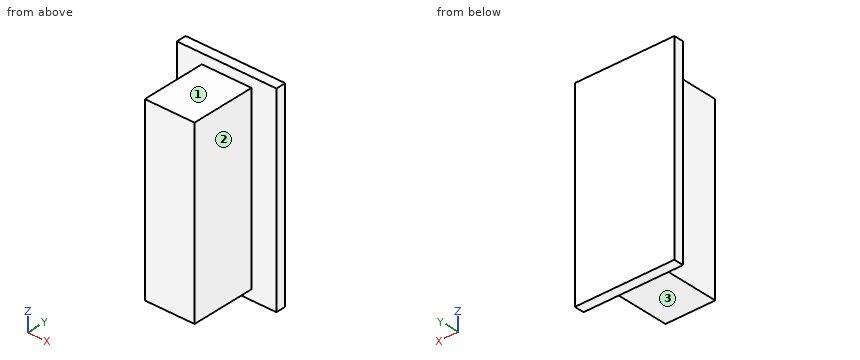
Autodesk Inventor part; units mm, degrees
ref_plane "YZ Plane" through (0, 0, 0) normal (1, 0, 0) x (0, 1, 0)
ref_plane "XZ Plane" through (0, 0, 0) normal (0, 1, 0) x (-1, 0, 0)
ref_plane "XY Plane" through (0, 0, 0) normal (0, 0, 1) x (1, 0, 0)
sketch "スケッチ1" plane through (0, 0, 0) normal (0, 1, 0) x (-1, 0, 0)
  line L0 (10, 20) -> (-10, 20)
  line L1 (-10, 20) -> (-10, -20)
  line L2 (-10, -20) -> (10, -20)
  line L3 (10, -20) -> (10, 20)
  line L4 (10, 20) -> (-10, -20) construction
  line L5 (-10, 20) -> (10, -20) construction
  line L6 (5, 18) -> (-5, 18)
  line L7 (-5, 18) -> (-5, -18)
  line L8 (-5, -18) -> (5, -18)
  line L9 (5, -18) -> (5, 18)
  line L10 (5, 18) -> (-5, -18) construction
  line L11 (-5, 18) -> (5, -18) construction
  point P0 (0, 0)
  dimension "d0" = 40
  dimension "d1" = 20
  dimension "d2" = 2
  dimension "d3" = 10
extrude "押し出し1" add sketch "スケッチ1" along normal blind 2 contours L3 L2 L1 L0 | L9 L8 L7 L6
extrude "押し出し2" add sketch "スケッチ1" against normal blind 13 contours L9 L8 L7 L6
properties part number "i2chub"
Check sheet for the modelled part. Datum: model origin and axes. Units: mm. Face numbers are marked on the shaded views. A direction names the side the tool comes from. Round coordinates to 2 decimals unless told otherwise and drop trailing zeros. Order: outer loops, then holes, each group sorted by start corner. A loop starts at its lowest first (then second) coordinate and runs counter-clockwise, first axis right, second up.
Q1. Cross-section at A-A, the plane x = 3.5. Enter the section's corners in (y, z), plus the area to 3 significant figures.
Filled sheet:
outline: (-13, -18) - (0, -18) - (0, -20) - (2, -20) - (2, 20) - (0, 20) - (0, 18) - (-13, 18) - close
area: 548 mm2
Q2. Depth check by flat-ended pin: P1, Ø4, axis at y = -8, z = -14, coming from the +X side; P2, Ø3, axis at y = -6.5, z = -0.5, coming from the -X side; P3, Ø5, axis at x = -0.5, y = -3.5, coming from the +Z side. Enter the tip coordinate at first touch or a pass-through.
Filled sheet:
P1: stops at x = 5
P2: stops at x = -5
P3: stops at z = 18
Q3. Set-up check for the marked faces 1, 2 and 3: record each of +Z, -Z, +X, -X, +Y, -Y from which the full face is reachable in a straight line by a thin tool's end or side.
Filled sheet:
face 1: +Z, +X, -X, -Y
face 2: +Z, -Z, +X, -Y
face 3: -Z, +X, -X, -Y
Q4. Scan lines: L1, parallel to X at y = -10, z = 14; L2, parallel to Z at x = 3.5, y = -3.5; L3, parallel to Y at x = -9, z = 3. Record each from-to range of solid material in increasing order.
Filled sheet:
L1: x = -5 to 5
L2: z = -18 to 18
L3: y = 0 to 2
Q5. Cross-section at C-C, the plane y = -4. Enter the section's corners in (x, z).
Filled sheet:
outline: (-5, -18) - (5, -18) - (5, 18) - (-5, 18) - close
Q6. Cross-section at B-B, the plane z = 7.5. Enter the section's corners in (x, y), plus the area to 3 significant figures.
Filled sheet:
outline: (-10, 0) - (-5, 0) - (-5, -13) - (5, -13) - (5, 0) - (10, 0) - (10, 2) - (-10, 2) - close
area: 170 mm2
Q7. Cross-section at D-D, the plane x = -7.25. Enter the section's corners in (y, z), plus the area to 3 significant figures.
Filled sheet:
outline: (0, -20) - (2, -20) - (2, 20) - (0, 20) - close
area: 80.0 mm2
